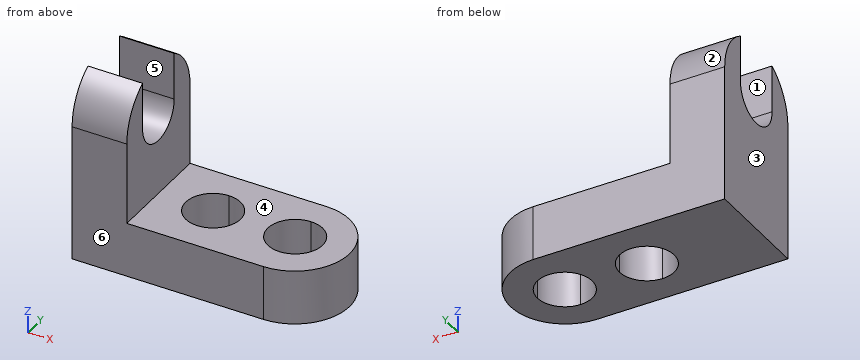
```python
from build123d import *

# Parameters (mm, degrees)
F1_DEPTH = 25.4
F3_DEPTH = 12.701
F5_DEPTH = 12.701


with BuildPart() as f1:
    # F0 (on Front) → F1 (new body)
    with BuildSketch(Plane.XZ):
        Polygon((0, 44.45), (0, 0), (57.15, 0), (57.15, 12.7), (12.7, 12.7), (12.7, 44.45), align=None)
    extrude(amount=F1_DEPTH)

    # F2 (on face) → F3 (cut, through all)
    with BuildSketch(Plane.XY.offset(12.7)):
        with BuildLine():
            Line((25.4, -19.05), (25.4, -6.35))
            ThreePointArc((25.4, -6.35), (19.05, -12.7), (25.4, -19.05))
        make_face()
        with BuildLine():
            ThreePointArc((31.75, -12.7), (29.8901280605, -8.2098719395), (25.4, -6.35))
            Line((25.4, -6.35), (25.4, -19.05))
            ThreePointArc((25.4, -19.05), (29.8901280605, -17.1901280605), (31.75, -12.7))
        make_face()
        with BuildLine():
            Line((44.45, -19.05), (44.45, -6.35))
            ThreePointArc((44.45, -6.35), (38.1, -12.7), (44.45, -19.05))
        make_face()
        with BuildLine():
            ThreePointArc((50.8, -12.7), (48.9401280605, -8.2098719395), (44.45, -6.35))
            Line((44.45, -6.35), (44.45, -19.05))
            ThreePointArc((44.45, -19.05), (48.9401280605, -17.1901280605), (50.8, -12.7))
        make_face()
        with BuildLine():
            Line((57.15, 0), (44.45, 0))
            ThreePointArc((44.45, 0), (57.0547872188, -12.7), (44.45, -25.4))
            Line((44.45, -25.4), (57.15, -25.4))
            Line((57.15, -25.4), (57.15, 0))
        make_face()
    extrude(amount=-F3_DEPTH, mode=Mode.SUBTRACT)

    # F4 (on face) → F5 (cut, through all)
    with BuildSketch(Plane.YZ.offset(12.7)):
        with BuildLine():
            Line((-25.4, 44.45), (-25.4, 31.75))
            ThreePointArc((-25.4, 31.75), (-23.6985226281, 38.1), (-19.05, 42.7485226281))
            Line((-19.05, 42.7485226281), (-19.05, 44.45))
            Line((-19.05, 44.45), (-25.4, 44.45))
        make_face()
        with BuildLine():
            ThreePointArc((-6.35, 42.7485226281), (-1.7014773719, 38.1), (0, 31.75))
            Line((0, 31.75), (0, 44.45))
            Line((0, 44.45), (-6.35, 44.45))
            Line((-6.35, 44.45), (-6.35, 42.7485226281))
        make_face()
        with BuildLine():
            ThreePointArc((-19.05, 31.75), (-12.7, 25.4), (-6.35, 31.75))
            Line((-6.35, 31.75), (-19.05, 31.75))
        make_face()
        with BuildLine():
            Line((-19.05, 31.75), (-6.35, 31.75))
            ThreePointArc((-6.35, 31.75), (-12.7, 38.1), (-19.05, 31.75))
        make_face()
        with BuildLine():
            ThreePointArc((-19.05, 31.75), (-12.7, 38.1), (-6.35, 31.75))
            Line((-6.35, 31.75), (-6.35, 42.7485226281))
            ThreePointArc((-6.35, 42.7485226281), (-9.4129981272, 44.0172579939), (-12.7, 44.45))
            ThreePointArc((-12.7, 44.45), (-15.9870018728, 44.0172579939), (-19.05, 42.7485226281))
            Line((-19.05, 42.7485226281), (-19.05, 31.75))
        make_face()
        with BuildLine():
            ThreePointArc((-12.7, 44.45), (-9.4129981272, 44.0172579939), (-6.35, 42.7485226281))
            Line((-6.35, 42.7485226281), (-6.35, 44.45))
            Line((-6.35, 44.45), (-12.7, 44.45))
        make_face()
        with BuildLine():
            Line((-19.05, 44.45), (-19.05, 42.7485226281))
            ThreePointArc((-19.05, 42.7485226281), (-15.9870018728, 44.0172579939), (-12.7, 44.45))
            Line((-12.7, 44.45), (-19.05, 44.45))
        make_face()
    extrude(amount=-F5_DEPTH, mode=Mode.SUBTRACT)


solid = f1.part
```
Can you work these out from the model? Positions are in its coordinate system, mm. Face numbers are marked on the shaded views. A direction names the side the tool comes from. Coordinates: 2 decimals unless noted, no trailing zeros. Order: outer loops, then holes, each group sorted by start corner. A loop starts at its lowest first (then second) coordinate and runs counter-clockwise, first axis right, second up. Notation, with made-up numbers: (-1, 83.25) -> (43, 83.25) arc R34 cw to (43, 115.25) -> close; hole circle Ø8 at (60.5, 49.25). An arc over 180 degrees is marked (long way). Write each question's results on one line, items separated by ' | '.
Item 1: I want a section at D-D, the plane x = 8. Write out the boundary of the cut face in (y, z).
Results are:
outline: (-25.4, 0) -> (0, 0) -> (0, 31.75) arc R12.7 ccw to (-6.35, 42.75) -> (-6.35, 31.75) arc R6.35 cw to (-19.05, 31.75) -> (-19.05, 42.75) arc R12.7 ccw to (-25.4, 31.75) -> close
Item 2: If we mould it in two halves opening along Y, with no side actions, what happens to the marked faces 1, 2 and 3? For each: +Y half, -Y half, draft (parallel to the pull), parting line (faces both ways), or undercut.
Results are:
face 1: undercut | face 2: +Y half | face 3: draft
Item 3: I'm going to push flat-ended pins straight in: pin 1 Ø10 at (x, z) = (51, 18) entering from +Y; pin 2 Ø12 at (y, z) = (-23, 18) entering from -X; pin 3 Ø4 at (y, z) = (-14.5, 24.5) entering from +X; pin 4 Ø3.5 at (x, z) = (3.5, 38.5) entering from -Y. Where does each tip first touch, or does it pass through?
Results are:
pin 1: through | pin 2: x = 0 | pin 3: x = 12.7 | pin 4: y = -24.37
Item 4: If I drill on line 1 along X through (y, z) = (-7, 19); line 2 along Y through (x, z) = (21, 12), over which ranges is the centre line in solid material (lowest first)?
Results are:
line 1: 0 to 12.7 | line 2: -25.4 to -17.28, -8.12 to 0
Item 5: I want a section at B-B, the plane y = -10.75. Write out the boundary of the cut face in (x, z).
Results are:
outline: (0, 0) -> (19.36, 0) -> (19.36, 12.7) -> (12.7, 12.7) -> (12.7, 25.71) -> (0, 25.71) -> close; (31.44, 0) -> (38.41, 0) -> (38.41, 12.7) -> (31.44, 12.7) -> close; (50.49, 0) -> (56.9, 0) -> (56.9, 12.7) -> (50.49, 12.7) -> close
Item 6: I want a section at A-A, the plane x = 45.5. Write out the boundary of the cut face in (y, z).
Results are:
outline: (-25.35, 0) -> (-18.96, 0) -> (-18.96, 12.7) -> (-25.35, 12.7) -> close; (-6.44, 0) -> (-0.05, 0) -> (-0.05, 12.7) -> (-6.44, 12.7) -> close
Item 7: I want a section at C-C, the plane z = 9.5. Write out the boundary of the cut face in (x, y), then the cut area to 3 significant figures.
Results are:
outline: (0, -25.4) -> (44.45, -25.4) arc R12.7 ccw to (44.45, 0) -> (0, 0) -> close; hole circle Ø12.7 at (25.4, -12.7); hole circle Ø12.7 at (44.45, -12.7) | area: 1,130 mm²
Item 8: Which directions (+Z, -Z, +X, -X, +Y, -Y) give clear straight access to the entire face, cutting with the end or side of a thin tool? Please do the marked faces 4, 5 and 6.
Results are:
face 4: +Z, +X, +Y, -Y | face 5: +Z, +X, -X | face 6: +Z, -Z, +X, -X, -Y
